Autodesk Inventor part; units mm, degrees
ref_plane "YZ Plane" through (0, 0, 0) normal (1, 0, 0) x (0, 1, 0)
ref_plane "XZ Plane" through (0, 0, 0) normal (0, 1, 0) x (-1, 0, 0)
ref_plane "XY Plane" through (0, 0, 0) normal (0, 0, 1) x (1, 0, 0)
sketch "Sketch1" plane through (0, 0, 0) normal (0, 0, 1) x (1, 0, 0)
  line L0 (-12.7, -12.7) -> (12.7, -12.7)
  line L1 (12.7, -12.7) -> (12.7, 12.7)
  line L2 (12.7, 12.7) -> (-12.7, 12.7)
  line L3 (-12.7, 12.7) -> (-12.7, -12.7)
  line L4 (-12.7, -12.7) -> (12.7, 12.7) construction
  line L5 (12.7, -12.7) -> (-12.7, 12.7) construction
  line L6 (-10.16, 10.16) -> (10.16, 10.16)
  line L7 (10.16, 10.16) -> (10.16, -10.16)
  line L8 (10.16, -10.16) -> (-10.16, -10.16)
  line L9 (-10.16, -10.16) -> (-10.16, 10.16)
  point P0 (0, 0)
  dimension "l1" = 25.4
  dimension "l2" = 25.4
  dimension "wt" = 2.54
extrude "Extrusion1" add sketch "Sketch1" against normal blind 152.4
sketch "Sketch2" plane through (-12.7, 12.7, 0) normal (0, 1, 0) x (1, 0, 0)
  line L0 (25.4, 0) -> (0, 0)
  line L1 (25.4, 0) -> (25.4, 152.4)
  line L2 (0, 152.4) -> (25.4, 152.4)
  line L3 (0, 0) -> (0, 152.4)
  point P0 (12.7, 0)
  point P1 (12.7, 12.7)
  dimension "d5" = 25.4
  dimension "d6" = 12.7
  dimension "d7" = 12.7
hole "Hole3" at (0, 12.7, -12.7) direction (0, -1, 0) diameter 4.0894 end through all
sketch "Sketch3" plane through (12.7, -12.7, 0) normal (1, 0, 0) x (0, 0, -1)
  line L0 (0, 0) -> (0, 25.4)
  line L1 (0, 0) -> (152.4, 0)
  line L2 (152.4, 25.4) -> (152.4, 0)
  line L3 (0, 25.4) -> (152.4, 25.4)
  point P0 (0, 12.7)
  point P1 (25.4, 12.7)
  dimension "d22" = 25.4
  dimension "d23" = 12.7
  dimension "d24" = 25.4
hole "Hole4" [suppressed]
pattern_linear "Rectangular Pattern1" count 7 spacing 25.4 along (0, 0, -1) of "Hole3"
pattern_linear "Rectangular Pattern2" [suppressed]
properties part number "versatubing_1x2x100" material "Aluminum 6061"
Design review of the part built by this model. Coordinates are the model's own, in mm. A direction names the side the tool comes from. Coordinates: 2 decimals unless noted, no trailing zeros. Loops run counter-clockwise (first coordinate to the right, second up) from the corner with the lowest first, then second, coordinate; pieces in that order, holes last.
Q1. To check wall thickness, follow line 1 (X direction, y = -11, z = -88.9); line 2 (Y direction, x = 7.5, z = -120). State the ranges of each line that lie inside material, in increasing order.
Reported:
line 1: x = -12.7 to -2.04, 2.04 to 12.7
line 2: y = -12.7 to -10.16, 10.16 to 12.7
Q2. Tool access review of faces 1 (the face through (-10.16, 0, -75)), 2 (the face through (0, 12.7, -75)): name each direction out of +Z, -Z, +X, -X, +Y, -Y from which nothing blocks a thin tool from reaching the whole face with its end or side.
Reported:
face 1: +Z, -Z
face 2: +Z, -Z, +X, -X, +Y
Q3. The part is to be moulded in two halves that separate along Y. For faces 3 (the face through (0, 10.16, -75)), 4 (the face through (-0.09, 11.412, -40.143)), 5 (the face through (0, -12.7, -75)), say which applies: +Y half, -Y half, draft (parallel to the pull), parting line (faces both ways), or undercut.
Reported:
face 3: undercut
face 4: draft
face 5: -Y half
Q4. We need section A-A on z = -88.9. State the section outline as (x, y) points, and give its area (3 significant figures).
Reported:
outline: (-12.7, -12.7) - (-2.04, -12.7) - (-2.04, -10.16) - (-10.16, -10.16) - (-10.16, 10.16) - (-2.04, 10.16) - (-2.04, 12.7) - (-12.7, 12.7) - close; (2.04, -12.7) - (12.7, -12.7) - (12.7, 12.7) - (2.04, 12.7) - (2.04, 10.16) - (10.16, 10.16) - (10.16, -10.16) - (2.04, -10.16) - close
area: 211 mm2
Q5. We need section B-B on y = -6.5. State the section outline as (x, z) points.
Reported:
outline: (-12.7, -152.4) - (-10.16, -152.4) - (-10.16, 0) - (-12.7, 0) - close; (10.16, -152.4) - (12.7, -152.4) - (12.7, 0) - (10.16, 0) - close
Q6. We need section D-D on z = -22.5. State the section outline as (x, y) points.
Reported:
outline: (-12.7, -12.7) - (12.7, -12.7) - (12.7, 12.7) - (-12.7, 12.7) - close; hole (-10.16, -10.16) - (10.16, -10.16) - (10.16, 10.16) - (-10.16, 10.16) - close
